```python
from build123d import *

# Parameters (mm, degrees)
SKETCH2_R           = 1.75
SKETCH2_R_2         = 7.5
FLANGE_DEPTH        = 15
SKETCH3_R           = 8.5
O_RING_SEAT_DEPTH   = 0.5
SKETCH5_R           = 1
OUTLET_DEPTH        = 27.561249971
BOSS_EXTRUDE2_REACH = 39.766
SKETCH6_R           = 3
SKETCH6_R_2         = 1


with BuildPart() as part:
    # Sketch2 → Flange (new body)
    with BuildSketch(Plane(origin=(0, 0, 0), x_dir=(0, 0, -1), z_dir=(1, 0, 0))):
        with BuildLine():
            ThreePointArc((-15.241152619, 2.820862781), (-15.5, 0), (-15.241152619, -2.820862781))
            ThreePointArc((-15.241152619, -2.820862781), (-13.297993041, -4.855781062), (-10.620697085, -5.721141055))
            ThreePointArc((-10.620697085, -5.721141055), (-7.247844507, -7.247844507), (-5.721141055, -10.620697085))
            ThreePointArc((-5.721141055, -10.620697085), (-4.855781062, -13.297993041), (-2.820862781, -15.241152619))
            ThreePointArc((-2.820862781, -15.241152619), (0, -15.5), (2.820862781, -15.241152619))
            ThreePointArc((2.820862781, -15.241152619), (4.855781062, -13.297993041), (5.721141055, -10.620697085))
            ThreePointArc((5.721141055, -10.620697085), (7.247844507, -7.247844507), (10.620697085, -5.721141055))
            ThreePointArc((10.620697085, -5.721141055), (13.297993041, -4.855781062), (15.241152619, -2.820862781))
            ThreePointArc((15.241152619, -2.820862781), (15.5, 0), (15.241152619, 2.820862781))
            ThreePointArc((15.241152619, 2.820862781), (13.297993041, 4.855781062), (10.620697085, 5.721141055))
            ThreePointArc((10.620697085, 5.721141055), (7.247844507, 7.247844507), (5.721141055, 10.620697085))
            ThreePointArc((5.721141055, 10.620697085), (4.855781062, 13.297993041), (2.820862781, 15.241152619))
            ThreePointArc((2.820862781, 15.241152619), (0, 15.5), (-2.820862781, 15.241152619))
            ThreePointArc((-2.820862781, 15.241152619), (-4.855781062, 13.297993041), (-5.721141055, 10.620697085))
            ThreePointArc((-5.721141055, 10.620697085), (-7.247844507, 7.247844507), (-10.620697085, 5.721141055))
            ThreePointArc((-10.620697085, 5.721141055), (-13.297993041, 4.855781062), (-15.241152619, 2.820862781))
        make_face()
        with Locations((0, 12)):
            Circle(SKETCH2_R, mode=Mode.SUBTRACT)
        with Locations((12, 0)):
            Circle(SKETCH2_R, mode=Mode.SUBTRACT)
        with Locations((0, -12)):
            Circle(SKETCH2_R, mode=Mode.SUBTRACT)
        with Locations((-12, 0)):
            Circle(SKETCH2_R, mode=Mode.SUBTRACT)
        Circle(SKETCH2_R_2, mode=Mode.SUBTRACT)
    extrude(amount=FLANGE_DEPTH)

    # Sketch3 → O-Ring Seat (cut)
    with BuildSketch(Plane(origin=(15, 0, 0), x_dir=(0, 0, -1), z_dir=(1, 0, 0))):
        Circle(SKETCH3_R)
    o_ring_seat = extrude(amount=-O_RING_SEAT_DEPTH, mode=Mode.SUBTRACT)

    # Mirror1: O-Ring Seat across plane
    add(o_ring_seat.mirror(Plane.ZY.offset(-7.5)), mode=Mode.SUBTRACT)

    # Sketch5 → Outlet (cut, through all)
    with BuildSketch(Plane(origin=(0, 0, 0), x_dir=(1, 0, 0), z_dir=(0, 1, 0))):
        with Locations(Location((7.5, 6.5, 0), (0, 0, 90))):
            Circle(SKETCH5_R)
    outlet = extrude(amount=OUTLET_DEPTH, mode=Mode.SUBTRACT)

    # Sketch6 → Boss-Extrude2 (add, up to next)
    with BuildSketch(Plane(origin=(0, 15.5, 0), x_dir=(1, 0, 0), z_dir=(0, 1, 0)), mode=Mode.PRIVATE) as boss_extrude2_sk1:
        with Locations(Location((7.5, 6.5, 0), (0, 0, 270))):
            Circle(SKETCH6_R)
        with Locations(Location((7.5, 6.5, 0), (0, 0, 90))):
            Circle(SKETCH6_R_2, mode=Mode.SUBTRACT)
    boss_extrude2_tool1 = extrude(boss_extrude2_sk1.sketch, amount=-BOSS_EXTRUDE2_REACH, mode=Mode.PRIVATE) - part.part
    boss_extrude2 = boss_extrude2_tool1.solids().sort_by_distance((7.5, 15.5, -9.415147))[0]
    add(boss_extrude2)

    # Inlet: Outlet, Boss-Extrude2 across plane
    add(outlet.mirror(Plane.XY), mode=Mode.SUBTRACT)
    add(boss_extrude2.mirror(Plane.XY))


solid = part.part
```
Read the model definition and answer for the solid it produces. Units are mm, in the model's axes. A direction names the side the tool comes from. Coordinates: 2 decimals unless noted, no trailing zeros. Write each loop counter-clockwise with the first axis right and the second up, starting at its lowest first coordinate (ties: lowest second). Pieces come first, ordered by that corner, then holes. Notation, with made-up numbers: (26, 58) -> (35, 58) arc R21 ccw to (35, 94) -> close; hole circle Ø6 at (-15.75, 24.5). An arc over 180 degrees is marked (long way). Return JSON: item names as keys, results as strings.
1. Find the intervals of material crossed by line 1 along Y through (x, z) = (4, 0); line 2 along Z through (x, y) = (1, -0.5); line 3 along X through (y, z) = (7.75, -6.5), in increasing order. Write a range as from..to.
Found:
{"line 1": "-15.5..-13.75, -10.25..-7.5, 7.5..10.25, 13.75..15.5", "line 2": "-15.49..-13.68, -10.32..-7.48, 7.48..10.32, 13.68..15.49", "line 3": "0..6.5, 8.5..15"}
2. A cutting plane is placed at C-C (z = 0). Determine the outline of the cut face in (x, y).
Found:
{"outline": "(0, -15.5) -> (15, -15.5) -> (15, -13.75) -> (0, -13.75) -> close; (0, -10.25) -> (15, -10.25) -> (15, -8.5) -> (14.5, -8.5) -> (14.5, -7.5) -> (0.5, -7.5) -> (0.5, -8.5) -> (0, -8.5) -> close; (0, 8.5) -> (0.5, 8.5) -> (0.5, 7.5) -> (14.5, 7.5) -> (14.5, 8.5) -> (15, 8.5) -> (15, 10.25) -> (0, 10.25) -> close; (0, 13.75) -> (15, 13.75) -> (15, 15.5) -> (0, 15.5) -> close"}
3. Determine the mould class of faces 3 (the face through (0.5, -8, 0)), 4 (the face through (7.4, 0, -15.5)), 5 (the face through (7.4, -15.5, 0)) for opening direction Z: pulls with the +Z half, pulls with the -Z half, needs draft (parallel to the pull), parting line crosses it, or undercut.
Found:
{"face 3": "undercut", "face 4": "pulls with the -Z half", "face 5": "parting line crosses it"}
4. A cutting plane is placed at A-A (y = 5). Determine the outline of the cut face in (x, z), and give its area (3 significant figures).
Found:
{"outline": "(0, -13.06) -> (15, -13.06) -> (15, -6.87) -> (14.5, -6.87) -> (14.5, -5.59) -> (7.91, -5.59) arc R1 cw (long way) to (7.09, -5.59) -> (0.5, -5.59) -> (0.5, -6.87) -> (0, -6.87) -> close; (0, 6.87) -> (0.5, 6.87) -> (0.5, 5.59) -> (7.09, 5.59) arc R1 cw (long way) to (7.91, 5.59) -> (14.5, 5.59) -> (14.5, 6.87) -> (15, 6.87) -> (15, 13.06) -> (0, 13.06) -> close", "area": "215 mm2"}
5. A cutting plane is placed at D-D (x = 2.75). Determine the outline of the cut face in (y, z).
Found:
{"outline": "(-15.24, -2.82) arc R5.73 ccw to (-10.62, -5.72) arc R5.25 cw to (-5.72, -10.62) arc R5.73 ccw to (-2.82, -15.24) arc R15.5 ccw to (2.82, -15.24) arc R5.73 ccw to (5.72, -10.62) arc R5.25 cw to (10.62, -5.72) arc R5.73 ccw to (15.24, -2.82) arc R15.5 ccw to (15.24, 2.82) arc R5.73 ccw to (10.62, 5.72) arc R5.25 cw to (5.72, 10.62) arc R5.73 ccw to (2.82, 15.24) arc R15.5 ccw to (-2.82, 15.24) arc R5.73 ccw to (-5.72, 10.62) arc R5.25 cw to (-10.62, 5.72) arc R5.73 ccw to (-15.24, 2.82) arc R15.5 ccw to start; hole circle Ø3.5 at (-12, 0); hole circle Ø15 at (0, 0); hole circle Ø3.5 at (0, -12); hole circle Ø3.5 at (0, 12); hole circle Ø3.5 at (12, 0)"}
6. A cutting plane is placed at B-B (x = 7.5). Give the number of separate pieces and of enclosed holes in the cut face, and give its area (3 significant figures).
Found:
{"separate pieces": "2", "enclosed holes": "4", "area": "369 mm2"}
7. A tool of negligible diameter and unlimited length cuts with its end or side. For faces 1 (the face through (7.4, -13.26, 4.88)), 2 (the face through (14.754, 7.167, -4.57)), from which of +Z, -Z, +X, -X, +Y, -Y can it reach the whole face along a straight path? Write none if from no direction.
Found:
{"face 1": "+Z, +X, -X, -Y", "face 2": "+X"}
8. Each of these flat-tipped pins is pushed along its axis until it touches: P1, Ø6, axis at x = 2.5, y = -7, coming from the -Z side; P2, Ø4.5, axis at y = -12, z = 0, coming from the -X side; P3, Ø2.5, axis at x = 7.5, z = -6.5, coming from the -Y side; P4, Ø12, axis at y = 0, z = 0, coming from the -X side. Where does it stop, or does it pass through?
Found:
{"P1": "z = -14.36", "P2": "x = 0", "P3": "y = -12.55", "P4": "through"}
